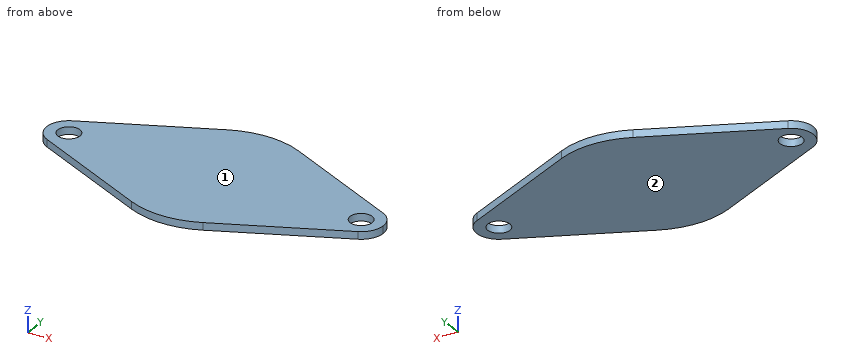
from build123d import *

# Parameters (mm, degrees)
F0_R     = 1.5
F0_R_2   = 8.5
F1_DEPTH = 1


with BuildPart() as f1:
    # F0 (on Top) → F1 (new body)
    with BuildSketch(Plane.XY):
        with BuildLine():
            ThreePointArc((-16.939914, 0.01004), (-18.331343, 2.542331), (-21.214914, 2.72562))
            ThreePointArc((-21.214914, 2.72562), (-22.939914, 0.01004), (-21.214914, -2.705541))
            ThreePointArc((-21.214914, -2.705541), (-18.331343, -2.522252), (-16.939914, 0.01004))
        make_face()
        with Locations((-19.939914, 0.01004)):
            Circle(F0_R, mode=Mode.SUBTRACT)
        with BuildLine():
            ThreePointArc((-4.827414, -10.399684), (-11.439914, 0.01004), (-4.827414, 10.419763))
            Line((-4.827414, 10.419763), (-21.214914, 2.72562))
            ThreePointArc((-21.214914, 2.72562), (-18.331343, 2.542331), (-16.939914, 0.01004))
            ThreePointArc((-16.939914, 0.01004), (-18.331343, -2.522252), (-21.214914, -2.705541))
            Line((-21.214914, -2.705541), (-4.827414, -10.399684))
        make_face()
        with BuildLine():
            ThreePointArc((4.947586, -10.399684), (9.767203, -6.156149), (11.560086, 0.01004))
            ThreePointArc((11.560086, 0.01004), (9.767203, 6.176228), (4.947586, 10.419763))
            ThreePointArc((4.947586, 10.419763), (0.060086, 11.51004), (-4.827414, 10.419763))
            ThreePointArc((-4.827414, 10.419763), (-11.439914, 0.01004), (-4.827414, -10.399684))
            ThreePointArc((-4.827414, -10.399684), (0.060086, -11.48996), (4.947586, -10.399684))
        make_face()
        with Locations((0.060086, 0.01004)):
            Circle(F0_R_2, mode=Mode.SUBTRACT)
        with Locations((0.060086, 0.01004)):
            Circle(F0_R_2)
        with BuildLine():
            ThreePointArc((4.947586, 10.419763), (9.767203, 6.176228), (11.560086, 0.01004))
            ThreePointArc((11.560086, 0.01004), (9.767203, -6.156149), (4.947586, -10.399684))
            Line((4.947586, -10.399684), (21.335086, -2.705541))
            ThreePointArc((21.335086, -2.705541), (17.060086, 0.01004), (21.335086, 2.72562))
            Line((21.335086, 2.72562), (4.947586, 10.419763))
        make_face()
        with BuildLine():
            ThreePointArc((23.060086, 0.01004), (22.592377, 1.61861), (21.335086, 2.72562))
            ThreePointArc((21.335086, 2.72562), (17.060086, 0.01004), (21.335086, -2.705541))
            ThreePointArc((21.335086, -2.705541), (22.592377, -1.598531), (23.060086, 0.01004))
        make_face()
        with Locations((20.060086, 0.01004)):
            Circle(F0_R, mode=Mode.SUBTRACT)
    extrude(amount=F1_DEPTH)


solid = f1.part
Can you work these out from the model? Positions are in its coordinate system, mm. Face numbers are marked on the shaded views. Give positions to 0.01 mm unless a question says otherwise; leave off trailing zeros. Loops run counter-clockwise (first coordinate to the right, second up) from the corner with the lowest first, then second, coordinate; pieces in that order, holes last. Notation, with made-up numbers: M 0.5,82.5 L 33.5,82.5 A23 cw 33.5,99.5 Z; hole C 36.25,62 d1. An arc over 180 degrees is marked long. One line per item, written item: value. Start each with the question number.
1) If we section it at A-A, the plane z = 0.6: Write out the boundary of the cut face in (x, y).
2) If we section it at B-B, the plane y = 0.5: Write out the boundary of the cut face in (x, z).
3) Thinking about a two-plate mould opening in Z: for the marked faces 1 and 2, which applies, +Z half, -Z half, draft (parallel to the pull), parting line (faces both ways), or undercut?
4) If I drill on line 1 (X direction, y = 1.25, z = 0.8); line 2 (Y direction, x = -21, z = 0.7); line 3 (X direction, y = 0.5, z = 0.2), over which ranges is the centre line in solid material (lowest first)? Write a range as [from, to].
5) If we section it at D-D, the plane x = 7: Write out the boundary of the cut face in (y, z), and give its area (3 significant figures).
6) If we section it at C-C, the plane y = 8.25: Write out the boundary of the cut face in (x, z).
Completed:
1. outline: M -21.21,-2.71 L -4.83,-10.4 A11.5 ccw 4.95,-10.4 L 21.34,-2.71 A3 ccw 23.06,0.01 A3 ccw 21.34,2.73 L 4.95,10.42 A11.5 ccw -4.83,10.42 L -21.21,2.73 A3 ccw Z; hole C -19.94,0.01 d3; hole C 20.06,0.01 d3
2. outline: M -22.9,0 L -21.36,0 L -21.36,1 L -22.9,1 Z; M -18.52,0 L 18.64,0 L 18.64,1 L -18.52,1 Z; M 21.48,0 L 23.02,0 L 23.02,1 L 21.48,1 Z
3. face 1: +Z half
3. face 2: -Z half
4. line 1: x = [-22.67, -20.78], [-19.1, 19.22], [20.9, 22.79]
4. line 2: y = [-2.81, -1.05], [1.07, 2.83]
4. line 3: x = [-22.9, -21.36], [-18.52, 18.64], [21.48, 23.02]
5. outline: M -9.44,0 L 9.46,0 L 9.46,1 L -9.44,1 Z
5. area: 18.9 mm^2
6. outline: M -9.45,0 L 9.57,0 L 9.57,1 L -9.45,1 Z
